from build123d import *

# Parameters (mm, degrees)
F0_W     = 24.411026
F0_H     = 21.652587
F1_DEPTH = 50
F2_SIZE  = 5


with BuildPart() as f1:
    # F0 (on Front) → F1 (new body)
    with BuildSketch(Plane.XZ):
        with Locations((-51.131187, 54.019387)):
            Rectangle(F0_W, F0_H)
    extrude(amount=F1_DEPTH)

    # F2
    f2_edges = [f1.edges().sort_by_distance(p)[0] for p in [
        (-63.3367, -25, 64.845681),
        (-63.3367, -25, 43.193094),
        (-63.3367, 0, 54.019388),
        (-63.3367, -50, 54.019388),
        (-38.925674, -25, 64.845681),
        (-51.131187, 0, 64.845681),
        (-51.131187, -50, 64.845681),
    ]]
    chamfer(f2_edges, length=F2_SIZE)


solid = f1.part
The model under review builds one solid part; all positions refer to its coordinate system, in mm. Round coordinates to 2 decimals unless told otherwise and drop trailing zeros. Loops run counter-clockwise (first coordinate to the right, second up) from the corner with the lowest first, then second, coordinate; pieces in that order, holes last. Notation, with made-up numbers: M 40.5,86.5 L 59.5,86.5 A10 cw 59.5,92.5 Z; hole C 41,86.25 d11. An arc over 180 degrees is marked long. Answer as a JSON object with one key per item and string values.
Item 1: We need section B-B, the plane z = 53.5. State the section outline as (x, y) points, and give its area (3 significant figures).
Check sheet entries:
{"outline": "M -63.34,-45 L -58.34,-50 L -38.93,-50 L -38.93,0 L -58.34,0 L -63.34,-5 Z", "area": "1,200 mm2"}
Item 2: We need section A-A, the plane y = -39. State the section outline as (x, z) points, and give its area (3 significant figures).
Check sheet entries:
{"outline": "M -63.34,48.19 L -58.34,43.19 L -38.93,43.19 L -38.93,59.85 L -43.93,64.85 L -58.34,64.85 L -63.34,59.85 Z", "area": "491 mm2"}
Item 3: Clearance check with flat-ended pins moving along their axes: P1, Ø2, axis at x = -48, z = 62.5, coming from the -Y side; P2, Ø8, axis at x = -42, z = 56, coming from the +Y side. State where each tip first meets the part, or that it passes through.
Check sheet entries:
{"P1": "y = -48.35", "P2": "y = 0"}
Item 4: We need section C-C, the plane x = -46. State the section outline as (y, z) points, and give its area (3 significant figures).
Check sheet entries:
{"outline": "M -50,43.19 L 0,43.19 L 0,59.85 L -5,64.85 L -45,64.85 L -50,59.85 Z", "area": "1,060 mm2"}
Item 5: For line 1 along Z through (x, y) = (-56.25, -2.5); line 2 along Z through (x, y) = (-61.75, -29); line 3 along X through (y, z) = (-3.5, 58.75), list the stretches that pass through material, from the lowest coordinate up.
Check sheet entries:
{"line 1": "43.19 to 62.35", "line 2": "46.61 to 61.43", "line 3": "-61.84 to -38.93"}
